Source: CAD feature listing. Evaluate the final solid. Frame: model axes, mm. A direction names the side the tool comes from. Round coordinates to 2 decimals unless told otherwise and drop trailing zeros. Loops run counter-clockwise (first coordinate to the right, second up) from the corner with the lowest first, then second, coordinate; pieces in that order, holes last. Notation, with made-up numbers: (7, 49.5) - (22, 49.5) arc R14 ccw to (22, 67.5) - close; hole circle Ø4 at (-33, 10.25). An arc over 180 degrees is marked (long way). Write item = value, one per line. Start each with the question number.
from build123d import *

# Parameters (mm, degrees)
SKETCH1_R               = 19.84375
BOSS_EXTRUDE1_DEPTH     = 3.175
F_1_4_20_TAPPED_HOLE1_D = 5.1054
F_10_32_TAPPED_HOLE1_D  = 4.0386
CUT_EXTRUDE1_DEPTH      = 57.13926808


with BuildPart() as part:
    # Sketch1 → Boss-Extrude1 (new body)
    with BuildSketch(Plane(origin=(0, -335.48880086, 998.033966912), x_dir=(1, 0, 0), z_dir=(0, -0.318629355, 0.947879388))):
        with BuildLine():
            Line((-88.9, 1035.868385599), (-88.9, 982.73222125))
            Line((-88.9, 982.73222125), (-27.49630657, 876.377904457))
            ThreePointArc((-27.49630657, 876.377904457), (0, 860.502904457), (27.49630657, 876.377904457))
            Line((27.49630657, 876.377904457), (88.9, 982.73222125))
            Line((88.9, 982.73222125), (88.9, 1035.868385599))
            Line((88.9, 1035.868385599), (-88.9, 1035.868385599))
        make_face()
        with Locations((0, 892.252904457)):
            Circle(SKETCH1_R, mode=Mode.SUBTRACT)
    extrude(amount=BOSS_EXTRUDE1_DEPTH)

    # 1/4-20 Tapped Hole1 (through all)
    with Locations(Plane(origin=(0, -336.500449063, 1001.043483969), x_dir=(1, 0, 0), z_dir=(0, -0.318629355, 0.947879388))):
        with Locations((82.55, 1029.518385599), (-82.55, 1029.518385599)):
            Hole(F_1_4_20_TAPPED_HOLE1_D / 2)

    # #10-32 Tapped Hole1 (through all)
    with Locations(Plane(origin=(0, -336.500449063, 1001.043483969), x_dir=(1, 0, 0), z_dir=(0, -0.318629355, 0.947879388))):
        with Locations((18.52177825, 873.731126207), (-18.52177825, 873.731126207), (-18.52177825, 910.774682707), (18.52177825, 910.774682707)):
            Hole(F_10_32_TAPPED_HOLE1_D / 2)

    # Sketch6 → Cut-Extrude1 (cut, through all)
    with BuildSketch(Plane(origin=(0, -335.48880086, 998.033966912), x_dir=(-1, 0, 0), z_dir=(0, 0.318629355, -0.947879388))):
        with BuildLine():
            Line((-41.090457195, 975.803721018), (-41.090457195, 1046.47326385))
            Line((-41.090457195, 1046.47326385), (41.0904572, 1046.47326385))
            Line((41.0904572, 1046.47326385), (41.090457191, 975.803721018))
            ThreePointArc((41.090457191, 975.803721018), (35.75087991, 962.91284113), (22.860000022, 957.57326385))
            Line((22.860000022, 957.57326385), (-22.860000028, 957.57326385))
            ThreePointArc((-22.860000028, 957.57326385), (-35.750879915, 962.91284113), (-41.090457195, 975.803721018))
        make_face()
    extrude(amount=-CUT_EXTRUDE1_DEPTH, mode=Mode.SUBTRACT)


solid = part.part
(1) Access query for faces 5 (the face through (-83.922, 641.912, 1328.238)), 6 (the face through (-35.89, 576.87, 1306.38)). Directions: +Z, -Z, +X, -X, +Y, -Y. A direction counts if a zero-diameter tool reaches every point of the face in a straight line with its end or side. Return the directions, or none.
(2) Cut plane C-C (y = 545.5). Output: boundary loops of the cut face in (x, z).
(3) Material intervals for line 1 along X through (y, z) = (639, 1326.5); line 2 along Z through (x, y) = (-79.5, 638.5); line 3 along Z through (x, y) = (2, 567), sorted ascending. Write a range as from..to.
(4) Pin query (flat end, axial travel): P1, Ø2, axis at x = 59.5, y = 597.5, coming from the +Z side; P2, Ø2, axis at x = 14, z = 1282, coming from the +Y side. Return the tip coordinate at first contact, or that it passes through.
(5) Mould query, pull axis X, two halves, no side actions, for faces 1 (the face through (-1.245, 563.429, 1303.554)), 2 (the face through (-0.47, 479.67, 1273.7)), 3 (the face through (-18.084, 490.336, 1277.286)), 4 (the face through (-58.628, 545.824, 1295.938)). Classes: +X half, -X half, draft (parallel to the pull), parting line (faces both ways), or undercut.
(6) Cut plane D-D (x = 70). Output: boundary loops of the cut face in (y, z).
(7) Cut plane A-A (y = 629). Output: boundary loops of the cut face in (x, z), and give its area (3 significant figures).
(8) Cut plane B-B (x = -8). Output: boundary loops of the cut face in (y, z).
Solution:
q1.face_5 = none
q1.face_6 = +Z, +Y
q2.outline = (-58.74, 1297.53) - (-58.13, 1294.18) - (58.13, 1294.18) - (58.74, 1297.53) - close
q3.line_1 = -88.9..-84.82, -80.28..-41.09, 41.09..80.28, 84.82..88.9
q3.line_2 = 1325.44..1328.79
q3.line_3 = 1301.41..1304.75
q4.P1 = 1315.34
q4.P2 = through
q5.face_1 = draft
q5.face_2 = parting line
q5.face_3 = undercut
q5.face_4 = -X half
q6.outline = (563.98, 1303.74) - (564.99, 1300.73) - (646.39, 1328.09) - (645.38, 1331.1) - close
q7.outline = (-88.9, 1322.25) - (-41.09, 1322.25) - (-41.09, 1325.6) - (-88.9, 1325.6) - close; (41.09, 1322.25) - (88.9, 1322.25) - (88.9, 1325.6) - (41.09, 1325.6) - close
q7.area = 320 mm^2
q8.outline = (480.12, 1275.55) - (481.14, 1272.54) - (493.05, 1276.55) - (492.03, 1279.56) - close; (526.46, 1291.13) - (527.47, 1288.12) - (572.18, 1303.14) - (571.16, 1306.15) - close
